Design review of the part shown in the three views and the two pictorial views. Dimensions are in mm from the part's minimum x, y and z. A direction names the side the tool comes from. Coordinates: 2 decimals unless noted, no trailing zeros. Order: outer loops, then holes, each group sorted by start corner. A loop starts at its lowest first (then second) coordinate and runs counter-clockwise, first axis right, second up. Notation, with made-up numbers: (87, -21) -> (145, -21) arc R19 ccw to (145, -11) -> close; hole circle Ø9 at (68.25, 39.5). An arc over 180 degrees is marked (long way). Write item = value, one per line. Start each with the question number.
1) Wall thickness on probe 1 along Z at (x, y) = (30, 24); probe 2 along Z at (x, y) = (19, 15.25); probe 3 along Y at (x, z) = (13.5, 21): over which ranges is each line inside the solid? List them lowest first. Write a range as [from, to].
2) Consider section C-C on y = 17.5. Give the boundary of the cut face in (x, z), and give its area (4 significant figures).
3) Machinability: for the marked faces 1 and 2, which of the approach directions +Z, -Z, +X, -X, +Y, -Y give a long, thin tool a straight path to every point of the face, cutting with its end or side? Answer none if there is none.
4) Consider section B-B on z = 30. Give the boundary of the cut face in (x, y).
5) Consider section D-D on x = 44. Give the boundary of the cut face in (y, z) (1 decimal).
6) Draft analysis for pull direction Z (two halves, no side actions). For the marked faces 3, 4 and 5, state which applies: +Z half, -Z half, draft (parallel to the pull), parting line (faces both ways), or undercut.
7) Insertion check: pin 1 Ø10 at (x, z) = (14, 15) entering from -Y; pin 2 Ø7.5 at (x, z) = (19, 10.95) entering from -Y; pin 3 Ø1.5 at (x, y) = (37, 57.5) entering from -Z (1 decimal); pin 4 Ø12 at (x, y) = (31.5, 44.5) entering from -Z. Each pin has a flat end and moves straight along its axis. Give the tip position at first contact, or say it passes through.
8) Consider section A-A on x = 30. Give the boundary of the cut face in (y, z).
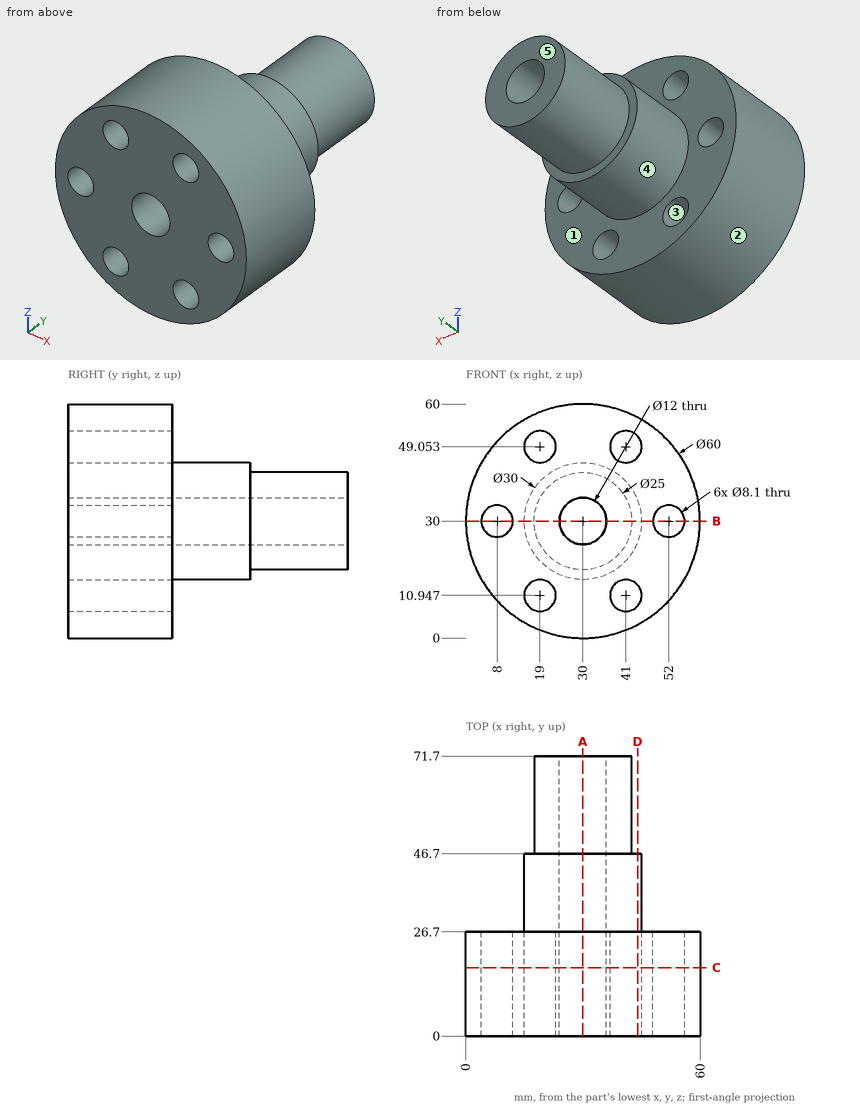
Answer sheet:
q1.probe_1 = [0, 24], [36, 60]
q1.probe_2 = [2.09, 6.9], [15, 45], [53.1, 57.91]
q1.probe_3 = [0, 26.7]
q2.outline = circle Ø60 at (30, 30); hole circle Ø8.1 at (8, 30); hole circle Ø8.1 at (19, 10.95); hole circle Ø8.1 at (19, 49.05); hole circle Ø12 at (30, 30); hole circle Ø8.1 at (41, 10.95); hole circle Ø8.1 at (41, 49.05); hole circle Ø8.1 at (52, 30)
q2.area = 2,405 mm2
q3.face_1 = +Y
q3.face_2 = +Y, -Y
q4.outline = (0, 0) -> (3.95, 0) -> (3.95, 26.7) -> (0, 26.7) -> close; (12.05, 0) -> (24, 0) -> (24, 71.7) -> (17.5, 71.7) -> (17.5, 46.7) -> (15, 46.7) -> (15, 26.7) -> (12.05, 26.7) -> close; (36, 0) -> (47.95, 0) -> (47.95, 26.7) -> (45, 26.7) -> (45, 46.7) -> (42.5, 46.7) -> (42.5, 71.7) -> (36, 71.7) -> close; (56.05, 0) -> (60, 0) -> (60, 26.7) -> (56.05, 26.7) -> close
q5.outline = (0, 3.5) -> (26.7, 3.5) -> (26.7, 8.2) -> (0, 8.2) -> close; (0, 13.7) -> (26.7, 13.7) -> (26.7, 24.6) -> (46.7, 24.6) -> (46.7, 35.4) -> (26.7, 35.4) -> (26.7, 46.3) -> (0, 46.3) -> close; (0, 51.8) -> (26.7, 51.8) -> (26.7, 56.5) -> (0, 56.5) -> close
q6.face_3 = undercut
q6.face_4 = parting line
q6.face_5 = draft
q7.pin_1 = 0
q7.pin_2 = through
q7.pin_3 = 19.2
q7.pin_4 = 15
q8.outline = (0, 0) -> (26.7, 0) -> (26.7, 15) -> (46.7, 15) -> (46.7, 17.5) -> (71.7, 17.5) -> (71.7, 24) -> (0, 24) -> close; (0, 36) -> (71.7, 36) -> (71.7, 42.5) -> (46.7, 42.5) -> (46.7, 45) -> (26.7, 45) -> (26.7, 60) -> (0, 60) -> close
